Autodesk Fusion 360 part; units mm, degrees
sketch "Szkic1" plane through (0, 0, 0) normal (0, 1, 0) x (1, 0, 0)
  line L0 (0, 0) -> (-50, 0) construction
  line L1 (-50, 0) -> (-50, -5) construction
  line L2 (-50, -5) -> (0, -5) construction
  line L3 (0, -5) -> (0, 0) construction
  line L4 (-3, -12) -> (-23.5581, -8.8372) construction
  line L5 (-3, -12) -> (0, -5) construction
  line L6 (-50, -5) -> (0, -5)
  line L7 (0, -5) -> (0, 0)
  line L8 (0, 0) -> (-50, 0)
  line L9 (-50, 0) -> (-50, -5)
  line L10 (-3, -12) -> (0, -5)
  line L11 (-3, -12) -> (-23.5581, -8.8372)
  line L12 (-23.5581, -8.8372) -> (-48.5, -5)
  line L13 (-23.5581, -8.8372) -> (-29.6404, -48.3721)
  line L14 (-3, -12) -> (-3.6082, -15.9535)
  line L15 (-6.9535, -11.3918) -> (-7.5617, -15.3453)
  line L16 (-7.5617, -15.3453) -> (-3.6082, -15.9535)
  line L17 (-29.6404, -48.3721) -> (-35.5706, -47.4597)
  line L18 (-35.5706, -47.4597) -> (-29.4884, -7.9249)
  line L19 (-7.5617, -15.3453) -> (-24.5594, -15.3453)
  dimension "d1" = 20.8
  dimension "d2" = 40
  dimension "d3" = 4
  dimension "d4" = 4
  dimension "d5" = 4
  dimension "d6" = 6
extrude "Wyciągnięcie proste1" add sketch "Szkic1" along normal blind 4
extrude "Wyciągnięcie proste2" add sketch "Szkic1" along normal blind 115 contours L6 L7 L8 L9 | L6 L10 L11 L12 | L12 L13 L17 L18 | L11 L14 L15 L16
extrude "Wyciągnięcie proste3" add sketch "Szkic1" along normal blind 4 from surface at 115
fillet "Zaokrąglenie1" radius 3 3 edges at (-50, 59.5, 5) (-48.5, 59.5, 5) (-29.4884, 59.5, 7.9249)
fillet "Zaokrąglenie2" radius 1 5 edges at (-16.0605, 0, 15.3453) (-5.585, 0, 15.6494) (-3.6082, 59.5, 15.9535) (-16.0605, 119, 15.3453) (-5.585, 119, 15.6494)
fillet "Zaokrąglenie3" radius 23 2 edges at (-3, 59.5, 12) (0, 59.5, 5)
Source: CAD feature listing. Evaluate the final solid. Frame: model axes, mm. A direction names the side the tool comes from. Coordinates: 2 decimals unless noted, no trailing zeros. Loops run counter-clockwise (first coordinate to the right, second up) from the corner with the lowest first, then second, coordinate; pieces in that order, holes last. Notation, with made-up numbers: (15, -14) - (26, -14) arc R37 cw to (26, 24) - close; hole circle Ø5 at (-31, 11.25). An arc over 180 degrees is marked (long way). Return JSON: item names as keys, results as strings.
Q1. Section C-C, the plane z = 28.5. Return loops of the section in (x, y).
Results:
{"outline": "(-32.65, 0) - (-26.58, 0) - (-26.58, 119) - (-32.65, 119) - close"}
Q2. Mould query, pull axis Z, two halves, no side actions, for faces 1 (the flat face through (-23, 0, 13)), 2 (the flat face through (-32.797, 58.667, 29.431)), 3 (the cylindrical face through (-2.813, 60.333, 12.012)). Classes: released by +Z, released by -Z, zero draft, split by the parting line, or undercut.
Results:
{"face 1": "zero draft", "face 2": "undercut", "face 3": "released by +Z"}
Q3. Section A-A, the plane x = -21.5. Return loops of the section in (y, z), plus the area to 3 significant figures.
Results:
{"outline": "(0, 0) - (119, 0) - (119, 14.35) arc R1 ccw to (118, 15.35) - (115, 15.35) - (115, 9.15) - (4, 9.15) - (4, 15.35) - (1, 15.35) arc R1 ccw to (0, 14.35) - close", "area": "1,140 mm2"}
Q4. Material intervals for line 1 along Z through (x, y) = (-20, 11); line 2 along X through (y, z) = (36, 46.5); line 3 along X through (y, z) = (8, 46), sorted ascending.
Results:
{"line 1": "0 to 9.38", "line 2": "-35.42 to -29.35", "line 3": "-35.35 to -29.28"}
Q5. Contact query for flat-ended pins moving along their axis: P1, Ø2, axis at y = 39, z = 5, coming from the +X side; P2, Ø1, axis at y = 13, z = 43, coming from the -X side; P3, Ø3, axis at y = 34.5, z = 42.5, coming from the +X side. Output: stop coordinate, or through.
Results:
{"P1": "x = -0.3", "P2": "x = -34.96", "P3": "x = -28.51"}
Q6. Section D-D, the plane x = -16. Return loops of the section in (y, z).
Results:
{"outline": "(0, 0) - (119, 0) - (119, 14.35) arc R1 ccw to (118, 15.35) - (115, 15.35) - (115, 10) - (4, 10) - (4, 15.35) - (1, 15.35) arc R1 ccw to (0, 14.35) - close"}
Q7. Access query for faces 4 (the flat face through (-16, 2, 15.345)), 5 (the flat face through (-7.253, 58.723, 13.341)), 6 (the flat face through (-26.557, 58.667, 28.328)). Directions: +Z, -Z, +X, -X, +Y, -Y. A direction counts if a zero-diameter tool reaches every point of the face in a straight line with its end or side. Return the directions, or none.
Results:
{"face 4": "+Z, +Y, -Y", "face 5": "none", "face 6": "+Z"}
Q8. Section B-B, the plane x = -34. Return loops of the section in (y, z), plus the area to 3 significant figures.
Results:
{"outline": "(0, 0) - (119, 0) - (119, 7.23) - (0, 7.23) - close; (0, 37.25) - (119, 37.25) - (119, 47.7) - (0, 47.7) - close", "area": "2,100 mm2"}
